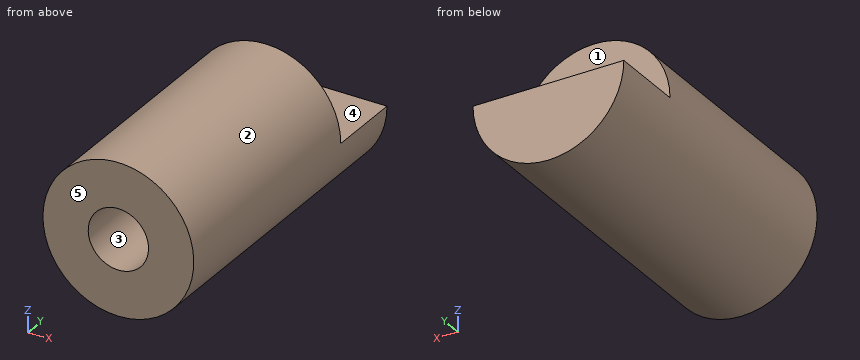
from build123d import *

# Parameters (mm, degrees)
SKETCH1_R                = 3.175
BOSS_EXTRUDE1_DEPTH      = 13.2715
SKETCH2_W                = 6.35
SKETCH2_H                = 4.534297592
CLEAR_LCD_FASTENER_DEPTH = 3.175
SKETCH3_R                = 1.27
TAP_NUMBER_4_DEPTH       = 8.509


with BuildPart() as part:
    # Sketch1 → Boss-Extrude1 (new body)
    with BuildSketch(Plane(origin=(0, 0, 0), x_dir=(1, 0, 0), z_dir=(0, 1, 0))):
        with Locations(Location((25.040432804, 11.35730315, 0), (0, 0, 90))):
            Circle(SKETCH1_R)
    extrude(amount=BOSS_EXTRUDE1_DEPTH)

    # Sketch2 → clear LCD fastener (cut)
    with BuildSketch(Plane(origin=(0, 13.2715, 0), x_dir=(1, 0, 0), z_dir=(0, 1, 0))):
        with Locations((25.040432804, 9.090154354)):
            Rectangle(SKETCH2_W, SKETCH2_H)
    extrude(amount=-CLEAR_LCD_FASTENER_DEPTH, mode=Mode.SUBTRACT)

    # Sketch3 → tap number 4 (cut)
    with BuildSketch(Plane.XZ):
        with Locations(Location((25.040432804, -11.35730315, 0), (0, 0, 270))):
            Circle(SKETCH3_R)
    extrude(amount=-TAP_NUMBER_4_DEPTH, mode=Mode.SUBTRACT)


solid = part.part
For this review, take the finished solid that the model builds, in its own axes (mm). Face numbers are marked on the shaded views. A direction names the side the tool comes from. Give positions to 0.01 mm unless a question says otherwise; leave off trailing zeros. Order: outer loops, then holes, each group sorted by start corner. A loop starts at its lowest first (then second) coordinate and runs counter-clockwise, first axis right, second up. Notation, with made-up numbers: (17, 38.25) - (57, 38.25) arc R27 ccw to (57, 65.25) - close; hole circle Ø4 at (-11.5, 25). An arc over 180 degrees is marked (long way). Answer as a JSON object with one key per item and string values. Group by question number.
Item 1: Take a section at D-D on y = 8.75. Give the boundary of the cut face in (x, z) (3 decimals), and give its area (3 significant figures).
Item 2: Machinability: for the marked faces 4 and 5, which of the approach directions +Z, -Z, +X, -X, +Y, -Y give a long, thin tool a straight path to every point of the face, cutting with its end or side? Answer none if there is none.
Item 3: Take a section at C-C on y = 2.25. Give the boundary of the cut face in (x, z) (3 decimals), and give its area (3 significant figures).
Item 4: Draft analysis for pull direction X (two halves, no side actions). For the marked faces 1, 2 and 3, state which applies: pulls with the +X half, pulls with the -X half, needs draft (parallel to the pull), parting line crosses it, or undercut.
Item 5: Clearance check with flat-ended pins moving along their axes: pin 1 Ø1.3 at (x, z) = (25, -11) entering from -Y; pin 2 Ø1.5 at (y, z) = (10.5, -9) entering from +X; pin 3 Ø2.5 at (x, y) = (25.5, 12) entering from +Z. State where each tip first meets the part, or that it passes through.
Item 6: Take a section at A-A on z = -10.75. Give the boundary of the cut face in (x, y).
Item 7: Wall thickness on line 1 along X through (y, z) = (4.5, -11.75); line 2 along Y through (x, z) = (27.5, -9.75); line 3 along Y through (x, z) = (25, -11.75): over which ranges is each line inside the solid? List them lowest first.
Item 8: Take a section at B-B on x = 22.75. Give the boundary of the cut face in (y, z).
Reported:
{
 "1": {"outline": "circle Ø6.35 at (25.04, -11.357)", "area": "31.7 mm^2"},
 "2": {"face 4": "+Z, +X, -X, +Y", "face 5": "+Z, -Z, +X, -X, -Y"},
 "3": {"outline": "circle Ø6.35 at (25.04, -11.357); hole circle Ø2.54 at (25.04, -11.357)", "area": "26.6 mm^2"},
 "4": {"face 1": "needs draft", "face 2": "parting line crosses it", "face 3": "undercut"},
 "5": {"pin 1": "y = 8.51", "pin 2": "x = 27.71", "pin 3": "z = -11.36"},
 "6": {"outline": "(21.92, 0) - (23.93, 0) - (23.93, 8.51) - (26.16, 8.51) - (26.16, 0) - (28.16, 0) - (28.16, 10.1) - (21.92, 10.1) - close"},
 "7": {"line 1": "21.89 to 23.83, 26.25 to 28.19", "line 2": "0 to 10.1", "line 3": "8.51 to 13.27"},
 "8": {"outline": "(0, -13.56) - (13.27, -13.56) - (13.27, -11.36) - (10.1, -11.36) - (10.1, -9.16) - (0, -9.16) - close"}
}
